Job drawing, mm, ordinate dimensions from the low corner. One solid piece. A direction names the side the tool comes from. Round coordinates to 2 decimals unless told otherwise and drop trailing zeros. Loops run counter-clockwise (first coordinate to the right, second up) from the corner with the lowest first, then second, coordinate; pieces in that order, holes last. Notation, with made-up numbers: M -28,78 L 4,78 A26 cw 4,94 Z; hole C 31.25,65.25 d2. An arc over 180 degrees is marked long. One line per item, written item: value.
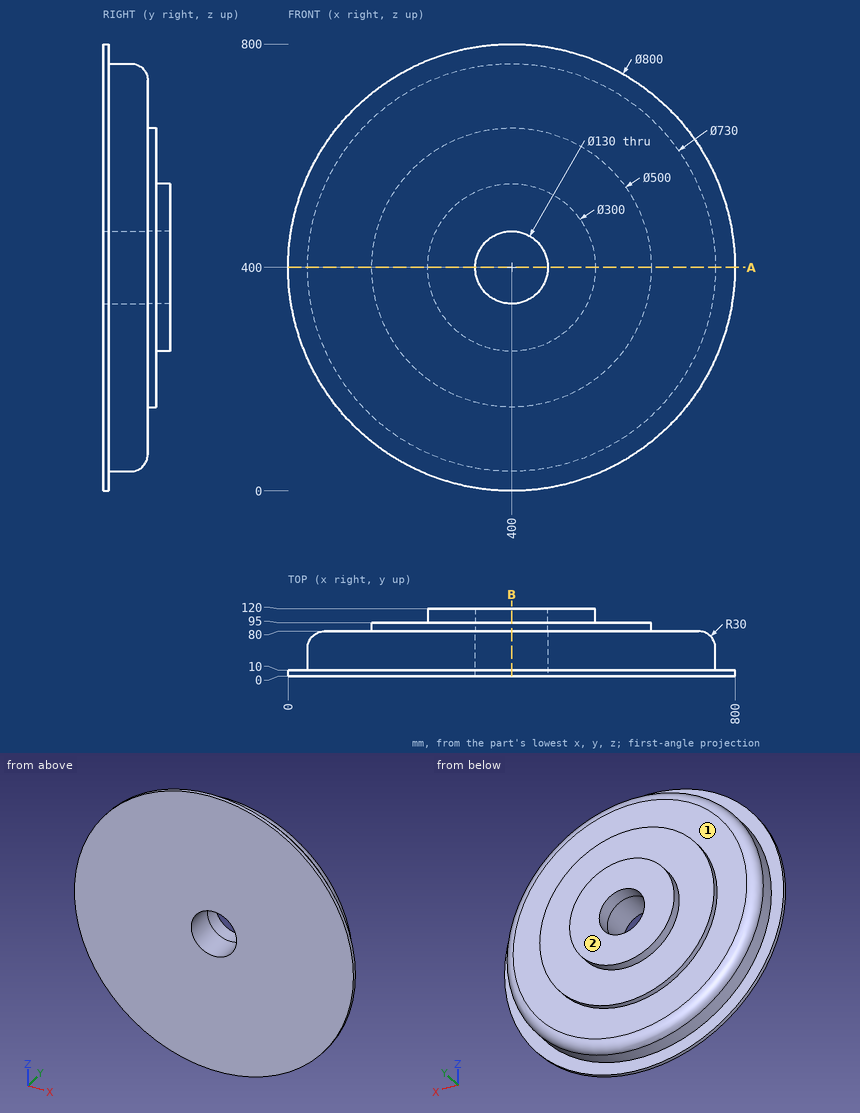
Item 1: Slice it at A-A, the plane z = 400. Give the cut face in (x, y).
Check values:
outline: M 0,0 L 335,0 L 335,120 L 250,120 L 250,95 L 150,95 L 150,80 L 65,80 A30 ccw 35,50 L 35,10 L 0,10 Z; M 465,0 L 800,0 L 800,10 L 765,10 L 765,50 A30 ccw 735,80 L 650,80 L 650,95 L 550,95 L 550,120 L 465,120 Z
Item 2: Drop flat-ended pins along their axis: P1, Ø5, axis at x = 137.5, z = 110, coming from the +Y side; P2, Ø12, axis at y = 74.5, z = 539.5, coming from the -X side; P3, Ø4, axis at x = 137, y = 30.5, coming from the +Z side. Give the stop position or say it passes through.
Check values:
P1: stops at y = 10
P2: stops at x = 69.06
P3: stops at z = 655.15
Item 3: Slice it at B-B, the plane x = 400. Give the cut face in (y, z), and give its area (3 significant figures).
Check values:
outline: M 0,0 L 10,0 L 10,35 L 50,35 A30 ccw 80,65 L 80,150 L 95,150 L 95,250 L 120,250 L 120,335 L 0,335 Z; M 0,465 L 120,465 L 120,550 L 95,550 L 95,650 L 80,650 L 80,735 A30 ccw 50,765 L 10,765 L 10,800 L 0,800 Z
area: 58,100 mm2
Item 4: Which spindle directions (+Z, -Z, +X, -X, +Y, -Y) get a long thin tool onto all of the face, cutting with end or side? Do the marked faces 1 and 2. Say none if no direction does.
Check values:
face 1: +Y
face 2: +Z, -Z, +X, -X, +Y
Item 5: Wall check: line 1 along Z through (x, y) = (400, 51); line 2 along Z through (x, y) = (400, 103.5); line 3 along X through (y, z) = (44, 400). Give the ranges that are in metal, low to high.
Check values:
line 1: z = 35.02 to 335, 465 to 764.98
line 2: z = 250 to 335, 465 to 550
line 3: x = 35 to 335, 465 to 765
